Read the model definition and answer for the solid it produces. Units are mm, in the model's axes. Face numbers are marked on the shaded views. A direction names the side the tool comes from. Coordinates: 2 decimals unless noted, no trailing zeros. Loops run counter-clockwise (first coordinate to the right, second up) from the corner with the lowest first, then second, coordinate; pieces in that order, holes last.
from build123d import *

# Parameters (mm, degrees)
BOSS_EXTRUDE1_DEPTH = 6
FILLET1_R           = 3


with BuildPart() as part:
    # Sketch1 → Boss-Extrude1 (new body)
    with BuildSketch(Plane(origin=(0, 0, 0), x_dir=(1, 0, 0), z_dir=(0, 1, 0))):
        with BuildLine():
            Line((0, 0), (23, 0))
            Line((23, 0), (23, 10))
            ThreePointArc((23, 10), (29, 16), (35, 10))
            Line((35, 10), (35, 0))
            Line((35, 0), (58, 0))
            Line((58, 0), (58, 20))
            Line((58, 20), (0, 20))
            Line((0, 20), (0, 0))
        make_face()
        with BuildLine():
            Line((9.705, 12.5), (9.705, 7.5))
            ThreePointArc((9.705, 7.5), (7.08, 4.875), (4.455, 7.5))
            Line((4.455, 7.5), (4.455, 12.5))
            ThreePointArc((4.455, 12.5), (7.08, 15.125), (9.705, 12.5))
        make_face(mode=Mode.SUBTRACT)
        with BuildLine():
            Line((48.295, 12.5), (48.295, 7.5))
            ThreePointArc((48.295, 7.5), (50.92, 4.875), (53.545, 7.5))
            Line((53.545, 7.5), (53.545, 12.5))
            ThreePointArc((53.545, 12.5), (50.92, 15.125), (48.295, 12.5))
        make_face(mode=Mode.SUBTRACT)
    extrude(amount=BOSS_EXTRUDE1_DEPTH)

    # Fillet1
    fillet1_edges = [part.edges().sort_by_distance(p)[0] for p in [
        (0, 3, -20),
        (58, 3, -20),
        (58, 3, 0),
        (0, 3, 0),
    ]]
    fillet(fillet1_edges, radius=FILLET1_R)


solid = part.part
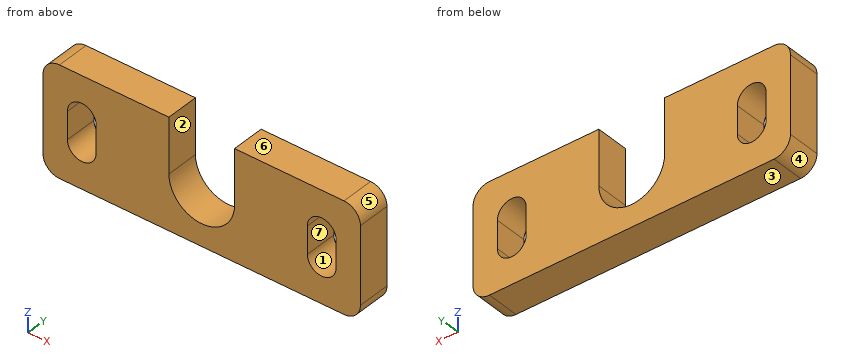
Item 1: Which of the six approach directions +Z, -Z, +X, -X, +Y, -Y give full straight-line access (tool end or side, diameter ignored) to the marked faces 1, 2 and 3?
Numbers:
face 1: +Y, -Y
face 2: +Z, +Y, -Y
face 3: -Z, +X, -X, +Y, -Y
Item 2: Determine the mould class of the marked faces 4, 5, 6 and 7 for opening direction X: released by +X, released by -X, zero draft, split by the parting line, or undercut.
Numbers:
face 4: released by -X
face 5: released by +X
face 6: zero draft
face 7: undercut
Item 3: Find the intervals of material crossed by line 1 along X through (y, z) = (2.4, -8.5) (3 decimals); line 2 along X through (y, z) = (1.65, -3.5); line 3 along X through (y, z) = (3.2, -14), in increasing order.
Numbers:
line 1: x = 0 to 4.455, 9.705 to 23, 35 to 48.295, 53.545 to 58
line 2: x = 0 to 23, 35 to 58
line 3: x = 0 to 4.93, 9.23 to 24.53, 33.47 to 48.77, 53.07 to 58
Item 4: A cutting plane is placed at D-D on z = -11. Determine the outline of the cut face in (x, y) (3 decimals).
Numbers:
outline: (0, 0) - (4.455, 0) - (4.455, 6) - (0, 6) - close; (9.705, 0) - (23.084, 0) - (23.084, 6) - (9.705, 6) - close; (34.916, 0) - (48.295, 0) - (48.295, 6) - (34.916, 6) - close; (53.545, 0) - (58, 0) - (58, 6) - (53.545, 6) - close
Item 5: A cutting plane is placed at B-B on y = 4.5. Determine the outline of the cut face in (x, z) (3 decimals).
Numbers:
outline: (0, -17) arc R3 ccw to (3, -20) - (55, -20) arc R3 ccw to (58, -17) - (58, -3) arc R3 ccw to (55, 0) - (35, 0) - (35, -10) arc R6 cw to (23, -10) - (23, 0) - (3, 0) arc R3 ccw to (0, -3) - close; hole (4.455, -12.5) arc R2.625 ccw to (9.705, -12.5) - (9.705, -7.5) arc R2.625 ccw to (4.455, -7.5) - close; hole (48.295, -12.5) arc R2.625 ccw to (53.545, -12.5) - (53.545, -7.5) arc R2.625 ccw to (48.295, -7.5) - close
Item 6: A cutting plane is placed at C-C on z = -8.75. Determine the outline of the cut face in (x, y) (3 decimals).
Numbers:
outline: (0, 0) - (4.455, 0) - (4.455, 6) - (0, 6) - close; (9.705, 0) - (23, 0) - (23, 6) - (9.705, 6) - close; (35, 0) - (48.295, 0) - (48.295, 6) - (35, 6) - close; (53.545, 0) - (58, 0) - (58, 6) - (53.545, 6) - close
Item 7: A cutting plane is placed at A-A on x = 7.08. Determine the outline of the cut face in (y, z) (3 decimals).
Numbers:
outline: (0, -20) - (6, -20) - (6, -15.125) - (0, -15.125) - close; (0, -4.875) - (6, -4.875) - (6, 0) - (0, 0) - close
Item 8: Given pin 1 (8 mm diameter, centred on x = 19.5, z = -5, fed in from -Y), flat-ended and moving along its own axis, determine where the tip first touches the part or whether it passes through.
Numbers:
pin 1: stops at y = 0
